Verification items for the finished model (mm, model axes). A direction names the side the tool comes from. Round coordinates to 2 decimals unless told otherwise and drop trailing zeros. Write each loop counter-clockwise with the first axis right and the second up, starting at its lowest first coordinate (ties: lowest second). Pieces come first, ordered by that corner, then holes. Notation, with made-up numbers: M 20,43 L 74,43 A6 ccw 74,54 Z; hole C -35.75,86 d2. An arc over 180 degrees is marked long. One line per item, written item: value. Start each with the question number.
Item 1: Section check B-B, the plane x = 2.75. Record the cut outline in (y, z).
Item 2: Section check C-C, the plane y = -2.5. Record the cut outline in (x, z).
Item 3: Tool access check on faces 1 (the face through (6.5, 4.2, -2.2)), 2 (the face through (0, 5.05, -13)), 3 (the face through (5, -5.05, -5)). Record the directions out of +Z, -Z, +X, -X, +Y, -Y that give a thin tool (end or side, any length) a straight path to the whole face; none if there is none.
Item 4: Thickness scan on probe 1 along Y at (x, z) = (3.5, -9.25); probe 2 along X at (y, z) = (-0.25, 4.5). Record the ranges inside material, lowest first. Write a range as from..to.
Item 5: Section check A-A, the plane z = -9.6. Record the cut outline in (x, y), then the cut area to 3 significant figures.
Item 6: Section check D-D, the plane y = -6. Record the cut outline in (x, z).
Item 7: Gauge pin test, flat ends, axial feed: pin 1 (9 mm diameter, centred on y = -1.5, z = -2.5, fed in from -X); pin 2 (1.2 mm diameter, centred on x = 6, z = -4.5, fed in from -Y); pin 3 (2.5 mm diameter, centred on x = 1, z = -11.5, fed in from +Y); pin 4 (8 mm diameter, centred on y = 2, z = -8.5, fed in from -X). Record the tip position at first contact, or that the pin passes through.
from build123d import *

# Parameters (mm, degrees)
SKETCH_2_W           = 23.6
SKETCH_2_H           = 16
EXTRUDE_1_DEPTH      = 4
EXTRUDE_START        = 4
EXTRUDE_3_DEPTH      = 4.5
SKETCH_5_R           = 0.3
CUT_EXTRUDE_10_DEPTH = 1
EXTRUDE_2_DEPTH      = 2.5
SKETCH_6_W           = 4
SKETCH_6_H           = 2.95
CUT_EXTRUDE_11_DEPTH = 10
SKETCH_7_R           = 0.3
CUT_EXTRUDE_12_DEPTH = 24.50132975
SKETCH_8_W           = 13.6
SKETCH_8_H           = 2.95
CUT_EXTRUDE_13_DEPTH = 2.5


with BuildPart() as part:
    # 草图2 → 凸台-拉伸1 (new body)
    with BuildSketch(Plane(origin=(0, 0, 0), x_dir=(0, 0, -1), z_dir=(1, 0, 0))):
        with Locations((5.8, 0)):
            Rectangle(SKETCH_2_W, SKETCH_2_H)
    extrude(amount=EXTRUDE_1_DEPTH)

    # 草图2<10> → 凸台-拉伸3 (add)
    with BuildSketch(Plane(origin=(0, 0, 0), x_dir=(0, 0, -1), z_dir=(1, 0, 0)).offset(EXTRUDE_START)):
        with BuildLine():
            ThreePointArc((0, -1.8), (1.272792206, -1.272792206), (1.8, 0))
            Line((1.8, 0), (0, 0))
            Line((0, 0), (0, -1.8))
        make_face()
        with BuildLine():
            Line((0, 0), (1.8, 0))
            ThreePointArc((1.8, 0), (1.272792206, 1.272792206), (0, 1.8))
            Line((0, 1.8), (0, 0))
        make_face()
        with BuildLine():
            Line((0, -1.8), (0, 0))
            Line((0, 0), (-1.8, 0))
            ThreePointArc((-1.8, 0), (-1.272792206, -1.272792206), (0, -1.8))
        make_face()
        with BuildLine():
            Line((-1.8, 0), (0, 0))
            Line((0, 0), (0, 1.8))
            ThreePointArc((0, 1.8), (-1.272792206, 1.272792206), (-1.8, 0))
        make_face()
    extrude(amount=EXTRUDE_3_DEPTH)

    # 草图5 → 切除-拉伸10 (cut)
    with BuildSketch(Plane(origin=(8.5, 0, 0), x_dir=(0, 0, -1), z_dir=(1, 0, 0))):
        Circle(SKETCH_5_R)
    extrude(amount=-CUT_EXTRUDE_10_DEPTH, mode=Mode.SUBTRACT)

    # 草图2<4> → 凸台-拉伸2 (add)
    with BuildSketch(Plane(origin=(0, 0, 0), x_dir=(0, 0, -1), z_dir=(1, 0, 0)).offset(EXTRUDE_START)):
        with BuildLine():
            ThreePointArc((-3.354101966, 3), (-1.837117307, 4.107919181), (0, 4.5))
            Line((0, 4.5), (-3.968626967, 4.5))
            ThreePointArc((-3.968626967, 4.5), (-4.643360347, 3.799895352), (-5.196152423, 3))
            Line((-5.196152423, 3), (-3.354101966, 3))
        make_face()
        with BuildLine():
            Line((0, 5), (1.8, 5))
            Line((1.8, 5), (1.8, 5.723635209))
            ThreePointArc((1.8, 5.723635209), (-1.245012655, 5.869407422), (-3.968626967, 4.5))
            Line((-3.968626967, 4.5), (0, 4.5))
            Line((0, 4.5), (0, 5))
        make_face()
        with BuildLine():
            ThreePointArc((0, 4.5), (0.919393397, 4.405078408), (1.8, 4.124318125))
            Line((1.8, 4.124318125), (1.8, 5))
            Line((1.8, 5), (0, 5))
            Line((0, 5), (0, 4.5))
        make_face()
        with BuildLine():
            ThreePointArc((1.8, 4.124318125), (3.764970119, 2.464751509), (4.5, 0))
            Line((4.5, 0), (6, 0))
            ThreePointArc((6, 0), (5.286764074, 2.837274331), (3.31662479, 5))
            Line((3.31662479, 5), (1.8, 5))
            Line((1.8, 5), (1.8, 4.124318125))
        make_face()
        with BuildLine():
            Line((1.8, 5.723635209), (1.8, 5))
            Line((1.8, 5), (3.31662479, 5))
            ThreePointArc((3.31662479, 5), (2.583771331, 5.415175501), (1.8, 5.723635209))
        make_face()
        with BuildLine():
            Line((6, 0), (4.5, 0))
            ThreePointArc((4.5, 0), (4.489038226, -0.313904132), (4.456206309, -0.626278954))
            Line((4.456206309, -0.626278954), (3.903880188, -4.556283516))
            ThreePointArc((3.903880188, -4.556283516), (5.262635021, -2.881782892), (5.941608412, -0.835038606))
            ThreePointArc((5.941608412, -0.835038606), (5.985384302, -0.418538842), (6, 0))
        make_face()
        with BuildLine():
            Line((5.356261262, -5), (5.941608412, -0.835038606))
            ThreePointArc((5.941608412, -0.835038606), (5.262635021, -2.881782892), (3.903880188, -4.556283516))
            Line((3.903880188, -4.556283516), (3.841519903, -5))
            Line((3.841519903, -5), (5.356261262, -5))
        make_face()
        Polygon((4.934638757, -8), (5.356261262, -5), (3.841519903, -5), (3.419897399, -8), align=None)
        with BuildLine():
            ThreePointArc((-5.196152423, 3), (-4.643360347, 3.799895352), (-3.968626967, 4.5))
            Line((-3.968626967, 4.5), (-6, 4.5))
            Line((-6, 4.5), (-6, 3))
            Line((-6, 3), (-5.196152423, 3))
        make_face()
    extrude(amount=EXTRUDE_2_DEPTH)

    # 草图6 → 切除-拉伸11 (cut)
    with BuildSketch(Plane(origin=(0, 0, -17.6), x_dir=(-1, 0, 0), z_dir=(0, 0, -1))):
        with Locations((-2, 6.525)):
            Rectangle(SKETCH_6_W, SKETCH_6_H)
        with Locations((-2, -6.525)):
            Rectangle(SKETCH_6_W, SKETCH_6_H)
    extrude(amount=-CUT_EXTRUDE_11_DEPTH, mode=Mode.SUBTRACT)

    # 草图7 → 切除-拉伸12 (cut, through all)
    with BuildSketch(Plane.XZ.offset(5.05)):
        with Locations((0, -9.6)):
            Circle(SKETCH_7_R)
        with Locations((0, -15.6)):
            Circle(SKETCH_7_R)
    extrude(amount=-CUT_EXTRUDE_12_DEPTH, mode=Mode.SUBTRACT)

    # 草图8 → 切除-拉伸13 (cut)
    with BuildSketch(Plane(origin=(6.5, 0, 0), x_dir=(0, 0, -1), z_dir=(1, 0, 0))):
        with Locations((0.8, -6.525)):
            Rectangle(SKETCH_8_W, SKETCH_8_H)
    extrude(amount=-CUT_EXTRUDE_13_DEPTH, mode=Mode.SUBTRACT)

    # 镜向1: part across plane


with BuildPart() as part_1:
    add(part.part)
    add(part.part.mirror(Plane(origin=(0, 0, 0), x_dir=(0, 0, 1), z_dir=(1, 0, 0))))


solid = part_1.part
Response values:
1. outline: M -8,-7.6 L -5.05,-7.6 L -5.05,-17.6 L 5.05,-17.6 L 5.05,-7.6 L 8,-7.6 L 8,6 L -8,6 Z
2. outline: M -6.5,-5.71 L -4,-5.71 L -4,-17.6 L 4,-17.6 L 4,-5.71 L 6.5,-5.71 L 6.5,-4.19 L 4,-4.19 L 4,6 L -4,6 L -4,-4.19 L -6.5,-4.19 Z; hole C 0,-15.6 d0.6; hole C 0,-9.6 d0.6
3. face 1: -Z, +X, +Y
3. face 2: -Z, +X, -X, +Y
3. face 3: +Z, -Z, +X, -Y
4. probe 1: y = -5.05..5.05
4. probe 2: x = -4..4
5. outline: M -4,-5.05 L -0.3,-5.05 L -0.3,5.05 L -4,5.05 Z; M 0.3,-5.05 L 4,-5.05 L 4,5.05 L 0.3,5.05 Z
5. area: 74.7 mm2
6. outline: M -4,-7.6 L 4,-7.6 L 4,6 L -4,6 Z
7. pin 1: stops at x = -8.5
7. pin 2: stops at y = -5.05
7. pin 3: stops at y = 5.05
7. pin 4: stops at x = -6.5
